```python
from build123d import *

# Parameters (mm, degrees)
SKETCH1_R           = 2.794
BOSS_EXTRUDE1_DEPTH = 5.08
SKETCH3_W           = 25.4
SKETCH3_H           = 11.43
BOSS_EXTRUDE2_DEPTH = 45.72
SKETCH4_W           = 22.096687199
SKETCH4_H           = 11.43
BOSS_EXTRUDE3_DEPTH = 12.7


with BuildPart() as part:
    # Sketch1 → Boss-Extrude1 (new body)
    with BuildSketch(Plane.XY):
        Polygon((-57.15, 2.54), (-57.15, -2.54), (-57.15, -5.715), (57.15, -5.715), (57.15, -2.54), (57.15, 2.54), (57.15, 5.715), (-57.15, 5.715), align=None)
        with Locations((50.8, 0)):
            Circle(SKETCH1_R, mode=Mode.SUBTRACT)
        with Locations((-50.8, 0)):
            Circle(SKETCH1_R, mode=Mode.SUBTRACT)
    extrude(amount=BOSS_EXTRUDE1_DEPTH)

    # Sketch3 → Boss-Extrude2 (add)
    with BuildSketch(Plane.XY.offset(5.08)):
        Rectangle(SKETCH3_W, SKETCH3_H)
    extrude(amount=BOSS_EXTRUDE2_DEPTH)

    # Sketch4 → Boss-Extrude3 (add)
    with BuildSketch(Plane.XY.offset(50.8)):
        with Locations((23.7483436, 0)):
            Rectangle(SKETCH4_W, SKETCH4_H)
        with Locations((-23.7483436, 0)):
            Rectangle(SKETCH4_W, SKETCH4_H)
    extrude(amount=-BOSS_EXTRUDE3_DEPTH)


solid = part.part
```
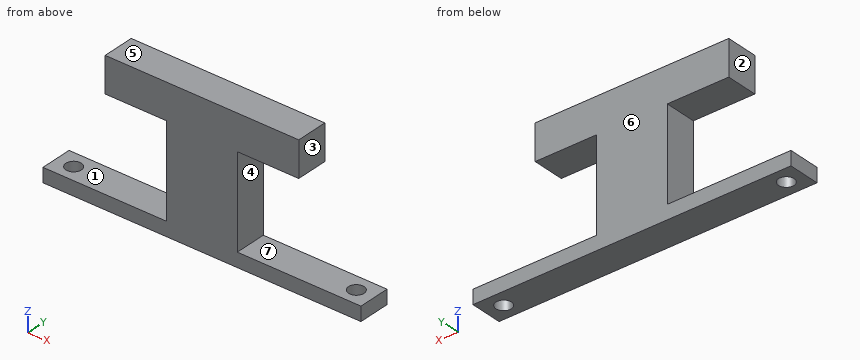
For this review, take the finished solid that the model builds, in its own axes (mm). Face numbers are marked on the shaded views. A direction names the side the tool comes from. Coordinates: 2 decimals unless noted, no trailing zeros. Write each loop counter-clockwise with the first axis right and the second up, starting at its lowest first coordinate (ties: lowest second). Pieces come first, ordered by that corner, then holes. Notation, with made-up numbers: (-24.75, 88) -> (-8.75, 88) arc R11 cw to (-8.75, 109) -> close; hole circle Ø6 at (-2, 81.5). An arc over 180 degrees is marked (long way). Put each result on its own line as item: value.
Q1. Tool access review of the marked faces 1, 2, 3 and 4: name each direction out of +Z, -Z, +X, -X, +Y, -Y from which nothing blocks a thin tool from reaching the whole face with its end or side.
From the geometry:
face 1: -X, +Y, -Y
face 2: +Z, -X, +Y, -Y
face 3: +Z, +X, +Y, -Y
face 4: +X, +Y, -Y
Q2. Take a section at B-B, the plane y = 1.75. State the section outline as (x, z) points.
From the geometry:
outline: (-57.15, 0) -> (-52.98, 0) -> (-52.98, 5.08) -> (-57.15, 5.08) -> close; (-48.62, 0) -> (48.62, 0) -> (48.62, 5.08) -> (12.7, 5.08) -> (12.7, 38.1) -> (34.8, 38.1) -> (34.8, 50.8) -> (-34.8, 50.8) -> (-34.8, 38.1) -> (-12.7, 38.1) -> (-12.7, 5.08) -> (-48.62, 5.08) -> close; (52.98, 0) -> (57.15, 0) -> (57.15, 5.08) -> (52.98, 5.08) -> close
Q3. Take a section at A-A, the plane x = -18.5. State the section outline as (y, z) points (3 decimals), then the cut area to 3 significant figures.
From the geometry:
outline: (-5.715, 0) -> (5.715, 0) -> (5.715, 5.08) -> (-5.715, 5.08) -> close; (-5.715, 38.1) -> (5.715, 38.1) -> (5.715, 50.8) -> (-5.715, 50.8) -> close
area: 203 mm2
Q4. Clearance check with flat-ended pins moving along their axes: pin 1 Ø3.5 at (x, y) = (-21.5, 0) entering from -Z; pin 2 Ø1 at (y, z) = (4, 33) entering from +X. State where each tip first meets the part, or that it passes through.
From the geometry:
pin 1: stops at z = 0
pin 2: stops at x = 12.7
Q5. Take a section at D-D, the plane z = 42. State the section outline as (x, y) points (3 decimals).
From the geometry:
outline: (-34.797, -5.715) -> (34.797, -5.715) -> (34.797, 5.715) -> (-34.797, 5.715) -> close
Q6. The part is to be moulded in two halves that separate along Z. For the marked faces 5, 6 and 7, say which applies: +Z half, -Z half, draft (parallel to the pull), parting line (faces both ways), or undercut.
From the geometry:
face 5: +Z half
face 6: draft
face 7: undercut
Q7. Take a section at C-C, the plane x = -50.8. State the section outline as (y, z) points (3 decimals), then the cut area to 3 significant figures.
From the geometry:
outline: (-5.715, 0) -> (-2.794, 0) -> (-2.794, 5.08) -> (-5.715, 5.08) -> close; (2.794, 0) -> (5.715, 0) -> (5.715, 5.08) -> (2.794, 5.08) -> close
area: 29.7 mm2
Q8. Wall thickness on L1, parallel to Z at x = 33.5, y = -2.25; L2, parallel to Y at x = 50.8, z = 3.2 (3 decimals); L3, parallel to X at y = 4.75, z = 33: over which ranges is each line inside the solid? List them lowest first.
From the geometry:
L1: z = 0 to 5.08, 38.1 to 50.8
L2: y = -5.715 to -2.794, 2.794 to 5.715
L3: x = -12.7 to 12.7
